Geometry: see drawing. Coordinates: mm, zero at the bounding-box minimum. A direction names the side the tool comes from. Give positions to 0.01 mm unless a question says otherwise; leave off trailing zeros. Order: outer loops, then holes, each group sorted by start corner. A loop starts at its lowest first (then second) coordinate and runs counter-clockwise, first axis right, second up. Notation, with made-up numbers: M -5,47 L 7,47 A26 cw 7,74 Z; hole C 70.5,81.5 d2. An arc over 180 degrees is marked long. Return JSON: item names as keys, results as strings.
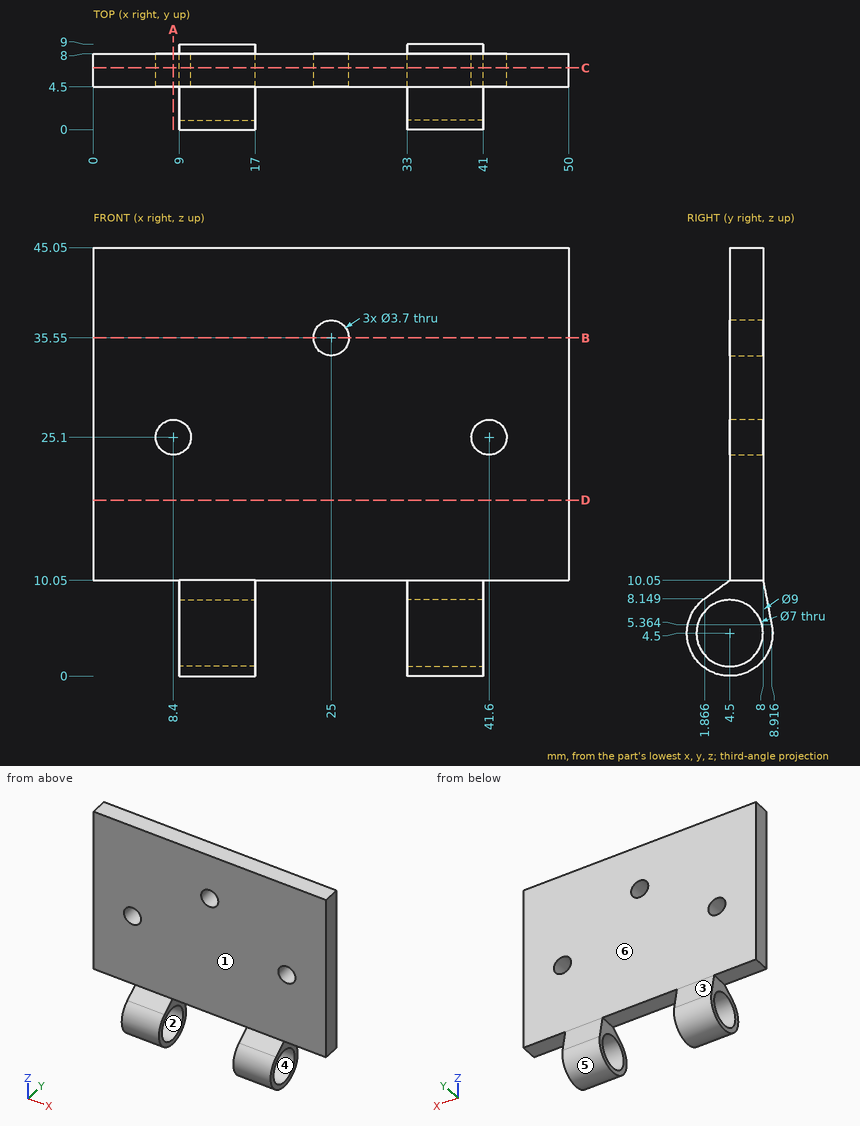
1. Section query D-D (z = 18.5). Return loops of the section in (x, y).
Evaluation:
{"outline": "M 0,4.5 L 50,4.5 L 50,8 L 0,8 Z"}
2. Section query A-A (x = 8.4). Return loops of the section in (y, z).
Evaluation:
{"outline": "M 4.5,10.05 L 8,10.05 L 8,23.25 L 4.5,23.25 Z; M 4.5,26.95 L 8,26.95 L 8,45.05 L 4.5,45.05 Z"}
3. Section query C-C (y = 6.5). Return loops of the section in (x, z), then the cut area to 3 significant figures.
Evaluation:
{"outline": "M 0,10.05 L 9,10.05 L 9,7.37 L 17,7.37 L 17,10.05 L 33,10.05 L 33,7.37 L 41,7.37 L 41,10.05 L 50,10.05 L 50,45.05 L 0,45.05 Z; M 9,0.47 L 17,0.47 L 17,1.63 L 9,1.63 Z; M 33,0.47 L 41,0.47 L 41,1.63 L 33,1.63 Z; hole C 8.4,25.1 d3.7; hole C 25,35.55 d3.7; hole C 41.6,25.1 d3.7", "area": "1,780 mm^2"}
4. First-contact query: pin 1 (1.5 mm diameter, centred on x = 31.5, z = 12, fed in from -Y); pin 2 (2 mm diameter, centred on x = 38.5, z = 11, fed in from +Y); pin 3 (4 mm diameter, centred on y = 4.5, z = 4.5, fed in from +X); pin 4 (3 mm diameter, centred on x = 3, y = 6.5, fed in from -Z). Flat tips, straight axial feed; report the tip coordinate or a pass-through.
Evaluation:
{"pin 1": "stops at y = 4.5", "pin 2": "stops at y = 8.01", "pin 3": "passes through", "pin 4": "stops at z = 10.05"}
5. Draft query along Y for the marked faces 1, 2, 3 and 4. Return one class per face: pulls with the +Y half, pulls with the -Y half, needs draft (parallel to the pull), parting line crosses it, or undercut.
Evaluation:
{"face 1": "pulls with the -Y half", "face 2": "undercut", "face 3": "pulls with the +Y half", "face 4": "undercut"}
6. Set-up query: the marked faces 5 and 6. Return all of +Z, -Z, +X, -X, +Y, -Y with unobstructed straight access to the full face (end or side cutting, diameter ignored); none if empty.
Evaluation:
{"face 5": "+X, -X", "face 6": "+Z, +X, -X, +Y"}
7. Section query B-B (z = 35.55). Return loops of the section in (x, y), then the cut area to 3 significant figures.
Evaluation:
{"outline": "M 0,4.5 L 23.15,4.5 L 23.15,8 L 0,8 Z; M 26.85,4.5 L 50,4.5 L 50,8 L 26.85,8 Z", "area": "162 mm^2"}
8. Ray query, probe 1 along X at (y, z) = (7.05, 25.1); probe 2 along X at (y, z) = (8, 5.5); probe 3 along Y at (x, z) = (37.5, 4.5). Return the intervals inside material, ascending.
Evaluation:
{"probe 1": "x = 0 to 6.55, 10.25 to 39.75, 43.45 to 50", "probe 2": "x = 9 to 17, 33 to 41", "probe 3": "y = 0 to 1, 8 to 9"}
